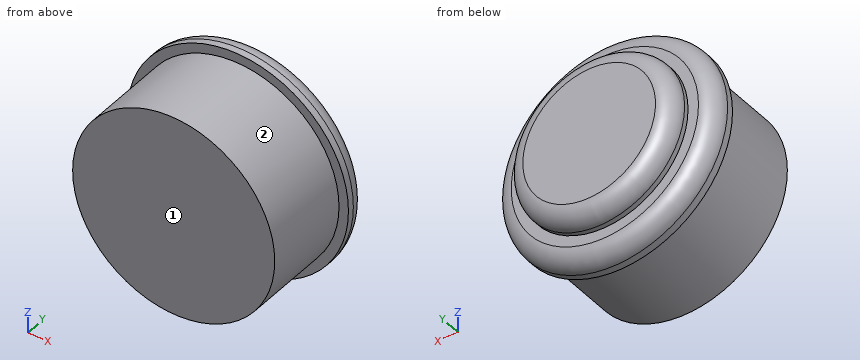
Autodesk Inventor part; units mm, degrees
ref_plane "YZ Plane" through (0, 0, 0) normal (1, 0, 0) x (0, 1, 0)
ref_plane "XZ Plane" through (0, 0, 0) normal (0, 1, 0) x (-1, 0, 0)
ref_plane "XY Plane" through (0, 0, 0) normal (0, 0, 1) x (1, 0, 0)
sketch "Sketch1" plane through (0, 0, 0) normal (0, 1, 0) x (-1, 0, 0)
  circle A0 centre (0, 0) radius 16.4
  dimension "d0" = 32.8
extrude "Extrusion1" add sketch "Sketch1" along normal blind 3.5
sketch "Sketch2" plane through (0, 3.5, 0) normal (0, 1, 0) x (1, 0, 0)
  circle A0 centre (0, 0) radius 12.35
  dimension "d3" = 24.7
extrude "Extrusion2" add sketch "Sketch2" along normal blind 3.2
fillet "Fillet1" radius 2.5 1 edges at (-12.35, 6.7, 0)
fillet "Fillet2" radius 2.5 1 edges at (16.4, 3.5, 0)
sketch "Sketch3" plane through (0, 0, 0) normal (0, -1, 0) x (1, 0, 0)
  circle A0 centre (0, 0) radius 15
  dimension "d8" = 30
extrude "Extrusion3" add sketch "Sketch3" along normal blind 13.1
properties part number "Large_button"
Here's how the part is built. I have some questions about the finished solid (model axes, mm). Face numbers are marked on the shaded views. Round coordinates to 2 decimals unless told otherwise and drop trailing zeros. Order: outer loops, then holes, each group sorted by start corner. A loop starts at its lowest first (then second) coordinate and runs counter-clockwise, first axis right, second up. Notation, with made-up numbers: M 41,79.5 L 66,79.5 A8 cw 66,87.5 Z; hole C -15,60.25 d2. An arc over 180 degrees is marked long. Answer in a Markdown table with one row per item.
Item 1: Imagine slicing it at C-C, the plane y = -5.5. Write out the boundary of the cut face in (x, z).
A:
| item | result |
|---|---|
| outline | C 0,0 d30 |
Item 2: Imagine slicing it at B-B, the plane x = 0. Write out the boundary of the cut face in (y, z).
A:
| item | result |
|---|---|
| outline | M -13.1,-15 L 0,-15 L 0,-16.4 L 1,-16.4 A2.5 ccw 3.5,-13.9 L 3.5,-12.35 L 4.2,-12.35 A2.5 ccw 6.7,-9.85 L 6.7,9.85 A2.5 ccw 4.2,12.35 L 3.5,12.35 L 3.5,13.9 A2.5 ccw 1,16.4 L 0,16.4 L 0,15 L -13.1,15 Z |
Item 3: I'm going to push flat-ended pins straight in: pin 1 (1.5 mm diameter, centred on y = -2, z = 3.5, fed in from -X); pin 2 (2 mm diameter, centred on x = 6, y = -4.5, fed in from +Z); pin 3 (5 mm diameter, centred on x = -1, y = -10, fed in from +Z). Where does each tip first touch, or does it pass through?
A:
| item | result |
|---|---|
| pin 1 | stops at x = -14.75 |
| pin 2 | stops at z = 14.14 |
| pin 3 | stops at z = 15 |
Item 4: If I drill on L1, parallel to Y at x = 4.5, z = -12; L2, parallel to Y at x = -12.5, z = 8.5; L3, parallel to Z at x = 5, y = -5.75, over which ranges is the centre line in solid material (lowest first)? Write a range as from..to.
A:
| item | result |
|---|---|
| L1 | y = -13.1..3.5 |
| L2 | y = 0..3.18 |
| L3 | z = -14.14..14.14 |
Item 5: Thinking about a two-plate mould opening in Z: for the marked faces 1 and 2, which applies, +Z half, -Z half, draft (parallel to the pull), parting line (faces both ways), or undercut?
A:
| item | result |
|---|---|
| face 1 | draft |
| face 2 | parting line |
Item 6: Imagine slicing it at A-A, the plane z = 0. Write out the boundary of the cut face in (x, y), and give its area (3 significant figures).
A:
| item | result |
|---|---|
| outline | M -16.4,0 L -15,0 L -15,-13.1 L 15,-13.1 L 15,0 L 16.4,0 L 16.4,1 A2.5 ccw 13.9,3.5 L 12.35,3.5 L 12.35,4.2 A2.5 ccw 9.85,6.7 L -9.85,6.7 A2.5 ccw -12.35,4.2 L -12.35,3.5 L -13.9,3.5 A2.5 ccw -16.4,1 Z |
| area | 581 mm2 |
